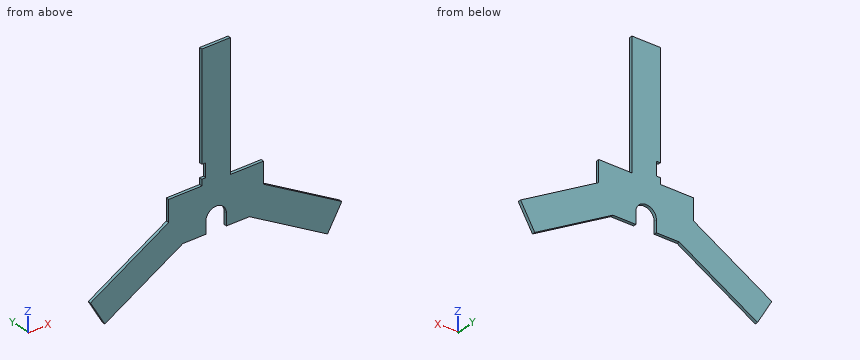
from build123d import *

# Parameters (mm, degrees)
SKETCH1_W           = 15.24
SKETCH1_H           = 19.327878735
SKETCH1_H_2         = 48.26
BOSS_EXTRUDE2_DEPTH = 1.5875
SKETCH6_W           = 2.032
SKETCH6_H           = 7.366
CUT_EXTRUDE4_DEPTH  = 2.54


with BuildPart() as part:
    # Sketch1 → Boss-Extrude2 (new body)
    with BuildSketch(Plane(origin=(0, 0, 0), x_dir=(1, 0, 0), z_dir=(0, 1, 0))):
        Polygon((50.8, 11.43), (0, 11.43), (0, 0), (17.78, 0), (33.02, 0), (50.8, 0), align=None)
        with BuildLine():
            Line((7.62, 24.628227154), (0, 11.43))
            Line((0, 11.43), (50.8, 11.43))
            Line((50.8, 11.43), (43.18, 24.628227154))
            Line((43.18, 24.628227154), (30.9, 24.628227154))
            Line((30.9, 24.628227154), (30.9, 18.264121265))
            ThreePointArc((30.9, 18.264121265), (25.4, 12.764121265), (19.9, 18.264121265))
            Line((19.9, 18.264121265), (19.9, 24.628227154))
            Line((19.9, 24.628227154), (7.62, 24.628227154))
        make_face()
        with Locations((25.4, -9.663939368)):
            Rectangle(SKETCH1_W, SKETCH1_H)
        Polygon((-41.794385987, 35.56), (-34.174385987, 48.758227154), (7.62, 24.628227154), (0, 11.43), align=None)
        with Locations((25.4, -43.457878735)):
            Rectangle(SKETCH1_W, SKETCH1_H_2)
        Polygon((84.974385987, 48.758227154), (92.594385987, 35.56), (50.8, 11.43), (43.18, 24.628227154), align=None)
    extrude(amount=BOSS_EXTRUDE2_DEPTH)

    # Sketch6 → Cut-Extrude4 (cut)
    with BuildSketch(Plane(origin=(0, 0, 0), x_dir=(-1, 0, 0), z_dir=(0, -1, 0))):
        with Locations((-18.796, -7.008878735)):
            Rectangle(SKETCH6_W, SKETCH6_H)
    extrude(amount=-CUT_EXTRUDE4_DEPTH, mode=Mode.SUBTRACT)


solid = part.part
Check sheet for the modelled part. Datum: model origin and axes. Units: mm. Round coordinates to 2 decimals unless told otherwise and drop trailing zeros. Order: outer loops, then holes, each group sorted by start corner. A loop starts at its lowest first (then second) coordinate and runs counter-clockwise, first axis right, second up.
Q1. Cross-section at B-B, the plane y = 0.95. Enter the section's corners in (x, z), plus the area to 3 significant figures.
Filled sheet:
outline: (-41.79, -35.56) - (-34.17, -48.76) - (7.62, -24.63) - (19.9, -24.63) - (19.9, -18.26) arc R5.5 cw to (30.9, -18.26) - (30.9, -24.63) - (43.18, -24.63) - (84.97, -48.76) - (92.59, -35.56) - (50.8, -11.43) - (50.8, 0) - (33.02, 0) - (33.02, 67.59) - (17.78, 67.59) - (17.78, 10.69) - (19.81, 10.69) - (19.81, 3.33) - (17.78, 3.33) - (17.78, 0) - (0, 0) - (0, -11.43) - close
area: 3,520 mm2
Q2. Cross-section at C-C, the plane x = 25.4. Enter the section's corners in (y, z), plus the area to 3 significant figures.
Filled sheet:
outline: (0, -12.76) - (1.59, -12.76) - (1.59, 67.59) - (0, 67.59) - close
area: 128 mm2
Q3. Scan lines: L1, parallel to X at y = 1.3, z = -8.5; L2, parallel to X at y = 0.5, z = 51.5; L3, parallel to Z at x = 18.5, y = 0.5. Record each from-to range of solid material in increasing order.
Filled sheet:
L1: x = 0 to 50.8
L2: x = 17.78 to 33.02
L3: z = -24.63 to 3.33, 10.69 to 67.59
Q4. Cross-section at A-A, the plane z = -30.5. Enter the section's corners in (x, y), plus the area to 3 significant figures.
Filled sheet:
outline: (-33.03, 0) - (-2.55, 0) - (-2.55, 1.59) - (-33.03, 1.59) - close; (53.35, 0) - (83.83, 0) - (83.83, 1.59) - (53.35, 1.59) - close
area: 96.8 mm2
Q5. Cross-section at D-D, the plane z = 56. Enter the section's corners in (x, y), plus the area to 3 significant figures.
Filled sheet:
outline: (17.78, 0) - (33.02, 0) - (33.02, 1.59) - (17.78, 1.59) - close
area: 24.2 mm2
Q6. Depth check by flat-ended pin: P1, Ø0.8, axis at y = 0.5, z = 38, coming from the +X side; P2, Ø0.8, axis at y = 1, z = 40.5, coming from the -X side; P3, Ø0.5, axis at y = 0.5, z = 6.5, coming from the -X side. Enter the tip coordinate at first touch or a pass-through.
Filled sheet:
P1: stops at x = 33.02
P2: stops at x = 17.78
P3: stops at x = 19.81
